```python
from build123d import *

# Parameters (mm, degrees)
F0_R         = 14.75
F1_DEPTH     = 30
F2_R         = 29.25
F3_DEPTH     = 19.5
F6_R         = 1
F8_W         = 73.76781106
F8_H         = 74.6486261487
F9_DEPTH     = 29.2510001
F10_T2_ANGLE = 183.7729101698
F11_R        = 1
F12_DEPTH    = 10


# Not quite as in the source:
# - a fillet or chamfer that OpenCascade refuses, or shapes differently, is made with other operations: its cross-section is extruded or revolved along the edge and cut away or added


with BuildPart() as f1:
    # F0 (on Top) → F1 (new body)
    with BuildSketch(Plane.XY):
        Circle(F0_R)
    extrude(amount=-F1_DEPTH)

    # F2 (on face) → F3 (join)
    with BuildSketch(Plane.XY):
        Circle(F2_R)
    extrude(amount=F3_DEPTH)

    # F4 (on Right) → F5 (revolve, cut)
    with BuildSketch(Plane.YZ):
        Polygon((13, 16.5), (13, 19.5), (0, 19.5), (0, -30), (10, -30), (10, -2.5), (11, 16.5), align=None)
    revolve(axis=Axis((0, 0, 5.2055120468), (0, 0, -1)), mode=Mode.SUBTRACT)

    # F6
    f6_edges = [f1.edges().sort_by_distance(p)[0] for p in [
        (-29.25, 0, 19.5),
        (0, -11, 16.5),
        (0, -13, 19.5),
        (0, -10, -30),
        (-14.75, 0, -30),
    ]]
    fillet(f6_edges, radius=F6_R)

    # F8 (on offset) → F9 (cut, through all)
    with BuildSketch(Plane.YZ):
        Rectangle(F8_W, F8_H)
    extrude(amount=-F9_DEPTH, mode=Mode.SUBTRACT)

    # F10: fillet of radius 5 on 1 edges, made by hand

    # F10_s1 → F10_t2 (revolve, cut)
    with BuildSketch(Plane(origin=(0, 0, 0), x_dir=(0, 0, 1), z_dir=(-0.999458026, -0.0329189041, 0))):
        with BuildLine():
            ThreePointArc((-2.6314879522, 10), (-2.5000454426, 10.0017280119), (-2.3686937866, 10.0069108533))
            Line((-2.3686937866, 10.0069108533), (-2.5, 10))
            Line((-2.5, 10), (-2.6314879522, 10))
        make_face()
    revolve(axis=Axis((0, 0, -2.5), (0, 0, -1)), revolution_arc=F10_T2_ANGLE, mode=Mode.SUBTRACT)

    # F11 (on face) → F12 (cut)
    with BuildSketch(Plane(origin=(0, 0, 0), x_dir=(0, -1, 0), z_dir=(-1, 0, 0))):
        with Locations((-21.587398374, 9.1951219512)):
            Circle(F11_R)
        with Locations((21.587398374, 9.1951219512)):
            Circle(F11_R)
    extrude(amount=-F12_DEPTH, mode=Mode.SUBTRACT)


solid = f1.part
```
Read the model definition and answer for the solid it produces. Units are mm, in the model's axes. A direction names the side the tool comes from. Coordinates: 2 decimals unless noted, no trailing zeros. Loops run counter-clockwise (first coordinate to the right, second up) from the corner with the lowest first, then second, coordinate; pieces in that order, holes last.
(1) The mould has two halves that part along Y. Classify faces 1 (the face through (17, 0, 19.5)), 2 (the face through (10, -22, 9)), 3 (the face through (14.746, -0.324, -14.297)), 4 (the face through (10, 0, -16)): released by +Y, released by -Y, zero draft, split by the parting line, or undercut.
Solution:
face 1: zero draft
face 2: undercut
face 3: split by the parting line
face 4: undercut
(2) The part is cut by section A-A (y = 0). Determine the outline of the cut face in (x, z).
Solution:
outline: (10, -29) arc R1 ccw to (11, -30) - (13.75, -30) arc R1 ccw to (14.75, -29) - (14.75, 0) - (29.25, 0) - (29.25, 18.5) arc R1 ccw to (28.25, 19.5) - (14, 19.5) arc R1 ccw to (13, 18.5) - (13, 16.5) - (11.95, 16.5) arc R1 ccw to (10.95, 15.55) - (10.01, -2.37) arc R5 ccw to (10, -2.63) - close
(3) The part is cut by section C-C (z = 14). Determine the outline of the cut face in (x, y), and give its area (3 significant figures).
Solution:
outline: (0, -29.25) arc R29.25 ccw to (0, 29.25) - (0, 10.87) arc R10.87 cw to (0, -10.87) - close
area: 1,160 mm2
(4) The part is cut by section B-B (z = -23.5). Determine the outline of the cut face in (x, y), and give its area (3 significant figures).
Solution:
outline: (0, -14.75) arc R14.75 ccw to (0, 14.75) - (0, 10) arc R10 cw to (0, -10) - close
area: 185 mm2
(5) Consider line 1 along Z through (x, y) = (4.5, -24); line 2 along Y through (x, z) = (5, 6); line 3 along Z through (x, y) = (6.25, -11). Determine where each line is inside the solid, lowest interval first.
Solution:
line 1: z = 0 to 19.5
line 2: y = -28.82 to -9.17, 9.17 to 28.82
line 3: z = -30 to 16.5
(6) A tool of negligible diameter and unlimited length cuts with its end or side. For faces 5 (the face through (4.93, 21.05, 10.04)), 6 (the face through (18, 0, 0)), 7 (the face through (29.243, -0.643, 9.12)), 8 (the face through (13, 0, 18)), from which of +Z, -Z, +X, -X, +Y, -Y can it reach the whole face along a straight path? Write none if from no direction.
Solution:
face 5: -X
face 6: -Z, +X
face 7: +Z, -Z, +X
face 8: +Z, -X
(7) Flat-ended cylindrical pins translate along their axes: pin 1 Ø1 at (y, z) = (21.5, 9.5) entering from -X; pin 2 Ø10 at (x, z) = (20.5, 5.5) entering from +Y; pin 3 Ø3 at (x, z) = (23, 3.5) entering from +Y; pin 4 Ø10 at (y, z) = (17.5, -12) entering from -X. Find the tip coordinate at first contact, or state that the pin passes through.
Solution:
pin 1: stops at x = 10
pin 2: stops at y = 24.81
pin 3: stops at y = 19.83
pin 4: stops at x = 0
